from build123d import *

# Parameters (mm, degrees)
SZKIC1_W                    = 96
SZKIC1_H                    = 39
DODANIE_WYCI_GNI_CIE1_DEPTH = 14
ZAOKR_GLENIE2_SIZE          = 3
ZAOKR_GLENIE2_SIZE_2        = 7
WYTNIJ_WYCI_GNI_CIE1_REACH  = 55.668
SZKIC3_R                    = 3.75
DODANIE_WYCI_GNI_CIE2_DEPTH = 10
DODANIE_WYCI_GNI_CIE3_DEPTH = 1.1
ZAOKR_GLENIE3_R             = 8
WYTNIJ_WYCI_GNI_CIE2_DEPTH  = 11
SZKIC6_W                    = 12.1
SZKIC6_H                    = 5.15
SZKIC6_W_2                  = 10.1
SZKIC6_H_2                  = 1.3
WYTNIJ_WYCI_GNI_CIE3_DEPTH  = 9.75
SZYK_LINIOWY1_COUNT         = 2
SZYK_LINIOWY1_PITCH         = 18.4
LUSTRO1_COPY_1_SKETCH_W     = 12.1
LUSTRO1_COPY_1_SKETCH_H     = 5.15
LUSTRO1_COPY_1_SKETCH_W_2   = 10.1
LUSTRO1_COPY_1_SKETCH_H_2   = 1.3
LUSTRO1_COPY_1_DEPTH        = 9.75
LUSTRO1_COPY_2_SKETCH_W     = 12.1
LUSTRO1_COPY_2_SKETCH_H     = 5.15
LUSTRO1_COPY_2_SKETCH_W_2   = 10.1
LUSTRO1_COPY_2_SKETCH_H_2   = 1.3
LUSTRO1_COPY_2_DEPTH        = 9.75


with BuildPart() as part:
    # Szkic1 → Dodanie-wyciągnięcie1 (new body)
    with BuildSketch(Plane(origin=(0, 0, 0), x_dir=(1, 0, 0), z_dir=(0, 1, 0))):
        Rectangle(SZKIC1_W, SZKIC1_H)
    extrude(amount=DODANIE_WYCI_GNI_CIE1_DEPTH)

    # Zaokrąglenie2
    # an asymmetric fillet: 7, 3 mm, written as the material it takes off along each edge
    with BuildSketch(Plane(origin=(65.5, 0, -19.5), x_dir=(0, 1, 0), z_dir=(-1, 0, 0)), Plane(origin=(-65.5, 0, 19.5), x_dir=(0, 1, 0), z_dir=(1, 0, 0))) as zaokr_glenie2_piece_1:
        with BuildLine():
            Bezier((ZAOKR_GLENIE2_SIZE, 0), (0, 0), (0, -ZAOKR_GLENIE2_SIZE_2), weights=[1, 0.707106781, 1])
            Line((0, -ZAOKR_GLENIE2_SIZE_2), (0, 0))
            Line((0, 0), (ZAOKR_GLENIE2_SIZE, 0))
        make_face()
    extrude(amount=131, mode=Mode.SUBTRACT)
    with BuildSketch(Plane(origin=(65.5, 14, -19.5), x_dir=(0, -1, 0), z_dir=(-1, 0, 0)), Plane(origin=(-65.5, 14, 19.5), x_dir=(0, -1, 0), z_dir=(1, 0, 0))) as zaokr_glenie2_piece_2:
        with BuildLine():
            Bezier((ZAOKR_GLENIE2_SIZE, 0), (0, 0), (0, ZAOKR_GLENIE2_SIZE_2), weights=[1, 0.707106781, 1])
            Line((0, ZAOKR_GLENIE2_SIZE_2), (0, 0))
            Line((0, 0), (ZAOKR_GLENIE2_SIZE, 0))
        make_face()
    extrude(amount=131, mode=Mode.SUBTRACT)

    # Wytnij-wyciągnięcie1: up to this face of the body (flat: up to its plane)
    wytnij_wyci_gni_cie1_end = Plane(part.part.faces().sort_by_distance((0, 0, 0))[0])
    # Szkic2 → Wytnij-wyciągnięcie1 (cut, up to the picked face)
    with BuildSketch(Plane(origin=(0, 14, 0), x_dir=(1, 0, 0), z_dir=(0, 1, 0)), mode=Mode.PRIVATE) as wytnij_wyci_gni_cie1_sk1:
        with BuildLine():
            Line((-48, -19.5), (-41, -19.5))
            ThreePointArc((-41, -19.5), (-45.949747468, -17.449747468), (-48, -12.5))
            Line((-48, -12.5), (-48, -19.5))
        make_face()
    wytnij_wyci_gni_cie1_tool1 = split(extrude(wytnij_wyci_gni_cie1_sk1.sketch, amount=-WYTNIJ_WYCI_GNI_CIE1_REACH, mode=Mode.PRIVATE), bisect_by=wytnij_wyci_gni_cie1_end, keep=Keep.BOTH, mode=Mode.PRIVATE)
    # Szkic2 → Wytnij-wyciągnięcie1 (cut, up to the picked face)
    with BuildSketch(Plane(origin=(0, 14, 0), x_dir=(1, 0, 0), z_dir=(0, 1, 0)), mode=Mode.PRIVATE) as wytnij_wyci_gni_cie1_sk2:
        with BuildLine():
            Line((-48, 19.5), (-41, 19.5))
            ThreePointArc((-41, 19.5), (-45.949747468, 17.449747468), (-48, 12.5))
            Line((-48, 12.5), (-48, 19.5))
        make_face()
    wytnij_wyci_gni_cie1_tool2 = split(extrude(wytnij_wyci_gni_cie1_sk2.sketch, amount=-WYTNIJ_WYCI_GNI_CIE1_REACH, mode=Mode.PRIVATE), bisect_by=wytnij_wyci_gni_cie1_end, keep=Keep.BOTH, mode=Mode.PRIVATE)
    # Szkic2 → Wytnij-wyciągnięcie1 (cut, up to the picked face)
    with BuildSketch(Plane(origin=(0, 14, 0), x_dir=(1, 0, 0), z_dir=(0, 1, 0)), mode=Mode.PRIVATE) as wytnij_wyci_gni_cie1_sk3:
        with BuildLine():
            Line((48, -19.5), (48, -12.5))
            ThreePointArc((48, -12.5), (45.949747468, -17.449747468), (41, -19.5))
            Line((41, -19.5), (48, -19.5))
        make_face()
    wytnij_wyci_gni_cie1_tool3 = split(extrude(wytnij_wyci_gni_cie1_sk3.sketch, amount=-WYTNIJ_WYCI_GNI_CIE1_REACH, mode=Mode.PRIVATE), bisect_by=wytnij_wyci_gni_cie1_end, keep=Keep.BOTH, mode=Mode.PRIVATE)
    # Szkic2 → Wytnij-wyciągnięcie1 (cut, up to the picked face)
    with BuildSketch(Plane(origin=(0, 14, 0), x_dir=(1, 0, 0), z_dir=(0, 1, 0)), mode=Mode.PRIVATE) as wytnij_wyci_gni_cie1_sk4:
        with BuildLine():
            Line((41, 19.5), (48, 19.5))
            Line((48, 19.5), (48, 12.5))
            ThreePointArc((48, 12.5), (45.949747468, 17.449747468), (41, 19.5))
        make_face()
    wytnij_wyci_gni_cie1_tool4 = split(extrude(wytnij_wyci_gni_cie1_sk4.sketch, amount=-WYTNIJ_WYCI_GNI_CIE1_REACH, mode=Mode.PRIVATE), bisect_by=wytnij_wyci_gni_cie1_end, keep=Keep.BOTH, mode=Mode.PRIVATE)
    add(wytnij_wyci_gni_cie1_tool1.solids().sort_by(Axis((-46.436424, 14, 17.936424), (0, -1, 0)))[0], mode=Mode.SUBTRACT)
    add(wytnij_wyci_gni_cie1_tool2.solids().sort_by(Axis((-46.436424, 14, -17.936424), (0, -1, 0)))[0], mode=Mode.SUBTRACT)
    add(wytnij_wyci_gni_cie1_tool3.solids().sort_by(Axis((46.436424, 14, 17.936424), (0, -1, 0)))[0], mode=Mode.SUBTRACT)
    add(wytnij_wyci_gni_cie1_tool4.solids().sort_by(Axis((46.436424, 14, -17.936424), (0, -1, 0)))[0], mode=Mode.SUBTRACT)

    # Szkic3 → Dodanie-wyciągnięcie2 (add)
    with BuildSketch(Plane(origin=(48, 0, 0), x_dir=(0, 0, -1), z_dir=(1, 0, 0))):
        with Locations(Location((0, 7, 0), (0, 0, 180))):
            Circle(SZKIC3_R)
    extrude(amount=DODANIE_WYCI_GNI_CIE2_DEPTH)

    # Szkic4 → Dodanie-wyciągnięcie3 (add)
    with BuildSketch(Plane.XZ):
        with BuildLine():
            Line((-48, 8.5), (-48, -8.5))
            ThreePointArc((-48, -8.5), (-39.5, 0), (-48, 8.5))
        make_face()
    extrude(amount=DODANIE_WYCI_GNI_CIE3_DEPTH)

    # Zaokrąglenie3
    # the kernel refuses this fillet: 8 mm, written as the material it takes off along each edge
    with BuildSketch(Plane(origin=(-48, -1.1, 0), x_dir=(-0.9293459551729958, 0, -0.36921009683321493), z_dir=(-0.36921009683321493, 0, 0.9293459551729958))) as zaokr_glenie3_piece_1:
        with BuildLine():
            CenterArc((4.451543504, -8), ZAOKR_GLENIE3_R, 59.598452337, 30.401547663)
            Line((4.451543504, 0), (4.451543504, 0.16))
            Line((4.451543504, 0.16), (8.5, 0.16))
            Line((8.5, 0.16), (8.66, 0))
            ThreePointArc((8.66, 0), (8.66, -0.55), (8.58096913, -0.962))
            Line((8.58096913, -0.962), (8.5, -1.1))
        make_face()
    revolve(axis=Axis((-48, -1.1, 0), (0, -1, 0)), revolution_arc=316.666179678, mode=Mode.SUBTRACT)

    # Szkic5 → Wytnij-wyciągnięcie2 (cut)
    with BuildSketch(Plane.ZY.offset(48)):
        Polygon((-5.875, 10.6), (5.875, 10.6), (5.875, 3.8), (3.15, 3.8), (3.15, 2.3), (1.65, 2.3), (1.65, 0.8), (-1.65, 0.8), (-1.65, 2.3), (-3.15, 2.3), (-3.15, 3.8), (-5.875, 3.8), align=None)
    extrude(amount=-WYTNIJ_WYCI_GNI_CIE2_DEPTH, mode=Mode.SUBTRACT)

    # Szkic6 → Wytnij-wyciągnięcie3 (cut)
    with BuildSketch(Plane.XY.offset(19.5)):
        with Locations((0, 7)):
            Rectangle(SZKIC6_W, SZKIC6_H)
        with Locations((0, 7.925)):
            Rectangle(SZKIC6_W_2, SZKIC6_H_2, mode=Mode.SUBTRACT)
    wytnij_wyci_gni_cie3 = extrude(amount=-WYTNIJ_WYCI_GNI_CIE3_DEPTH, mode=Mode.SUBTRACT)

    # Szyk liniowy1: Wytnij-wyciągnięcie3 ×2
    with Locations(*[(-i * SZYK_LINIOWY1_PITCH, 0, 0) for i in range(1, SZYK_LINIOWY1_COUNT)]):
        add(wytnij_wyci_gni_cie3, mode=Mode.SUBTRACT)

    # Lustro1 copy 1 sketch → Lustro1 copy 1 (cut)
    with BuildSketch(Plane(origin=(18.4, 0, 19.5), x_dir=(-1, 0, 0), z_dir=(0, 0, 1))):
        with Locations((0, -7)):
            Rectangle(LUSTRO1_COPY_1_SKETCH_W, LUSTRO1_COPY_1_SKETCH_H)
        with Locations((0, -7.925)):
            Rectangle(LUSTRO1_COPY_1_SKETCH_W_2, LUSTRO1_COPY_1_SKETCH_H_2, mode=Mode.SUBTRACT)
    extrude(amount=-LUSTRO1_COPY_1_DEPTH, mode=Mode.SUBTRACT)

    # Lustro1 copy 2 sketch → Lustro1 copy 2 (cut)
    with BuildSketch(Plane(origin=(0, 0, 19.5), x_dir=(-1, 0, 0), z_dir=(0, 0, 1))):
        with Locations((0, -7)):
            Rectangle(LUSTRO1_COPY_2_SKETCH_W, LUSTRO1_COPY_2_SKETCH_H)
        with Locations((0, -7.925)):
            Rectangle(LUSTRO1_COPY_2_SKETCH_W_2, LUSTRO1_COPY_2_SKETCH_H_2, mode=Mode.SUBTRACT)
    extrude(amount=-LUSTRO1_COPY_2_DEPTH, mode=Mode.SUBTRACT)


solid = part.part
Work out the finished part from the listing and answer in its coordinate system (mm). A direction names the side the tool comes from. Coordinates: 2 decimals unless noted, no trailing zeros. Put each result on its own line as item: value. Start each with the question number.
1) For a pull along X with two mould halves and no side action, classify faces 4 (the flat face through (-6.05, 7, 15)), 5 (the cylindrical face through (-45.9, 7.1, -17.5)), 6 (the cylindrical face through (46, 7.1, -17.4)) as released by +X, released by -X, zero draft, split by the parting line, or undercut.
2) Find section A-A (z = 14). State how many separate pieces and enclosed holes the cut face has, plus the area to 3 significant figures.
3) Flat-ended cylindrical pins translate along their axes: pin 1 (6 mm diameter, centred on y = 1.5, z = -14.5, fed in from +X); pin 2 (1.5 mm diameter, centred on x = -7.5, z = -6, fed in from -Y); pin 3 (2 mm diameter, centred on y = 6.5, z = -0.5, fed in from -X). Find the tip coordinate at first contact, or state that the pin passes through.
4) Find the intervals of material crossed by line 1 (X direction, y = 5.75, z = 12); line 2 (Y direction, x = 5, z = -10); line 3 (X direction, y = 8.5, z = -1.5), in increasing order. Write a range as from..to.
5) For faces 1 (the flat face through (0, 9.575, 15)), 2 (the cylindrical face through (52.93, 10.66, -0.81)), 3 (the flat face through (-43, 3.8, 5)), determine the directions among +Z, -Z, +X, -X, +Y, -Y from which every point of the face is accessible in a straight line to the end or side of a thin tool.
Results list:
1. face 4: undercut
1. face 5: released by -X
1. face 6: released by +X
2. separate pieces: 4
2. enclosed holes: 3
2. area: 1,180 mm^2
3. pin 1: stops at x = 48
3. pin 2: stops at y = 0
3. pin 3: stops at x = -37
4. line 1: x = -48..-24.45, -12.35..-6.05, 6.05..12.35, 24.45..48
4. line 2: y = 0..14
4. line 3: x = -37..58
5. face 1: +Z
5. face 2: +X
5. face 3: -X
